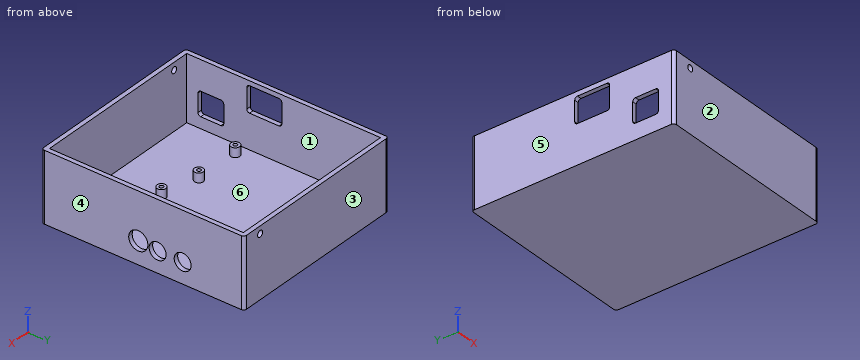
```python
from build123d import *

# Parameters (mm, degrees)
FLOOR_2P4MM_DEPTH                         = 2.4
SIX_PCB_SUPPORTS_5MM_START                = 2.4
SKETCH_2_R                                = 2.4
SIX_PCB_SUPPORTS_5MM_DEPTH                = 5
INTEGRAL_FRONT_REAR_AND_SIDE_WALLS_START  = 2.4
SKETCH_3_W                                = 94.1
SKETCH_3_H                                = 105.2
INTEGRAL_FRONT_REAR_AND_SIDE_WALLS_DEPTH  = 35.2
SIX_BLIND_M2P5_STANDOFF_PILOTS_DEPTH      = 2.05
SIX_BLIND_M2P5_STANDOFF_PILOTS_DEPTH_BACK = 2.05
SIX_BLIND_M2P5_STANDOFF_PILOTS_START      = 5.35
SKETCH_4_R                                = 1.05
SIDE_LID_SCREW_1_DEPTH                    = 1.25
SIDE_LID_SCREW_1_DEPTH_BACK               = 1.25
SIDE_LID_SCREW_1_START                    = -8.3
SKETCH_5_R                                = 1.7
SIDE_LID_SCREW_2_DEPTH                    = 1.25
SIDE_LID_SCREW_2_DEPTH_BACK               = 1.25
SIDE_LID_SCREW_2_START                    = 99.3
SKETCH_6_R                                = 1.7
FRONT_AUDIO_ACCESS_DEPTH                  = 1.25
FRONT_AUDIO_ACCESS_DEPTH_BACK             = 1.25
FRONT_AUDIO_ACCESS_START                  = 93.7
SKETCH_7_R                                = 5.2
SKETCH_7_R_2                              = 4.6
REAR_DC_AND_USB_ACCESS_DEPTH              = 1.25
REAR_DC_AND_USB_ACCESS_DEPTH_BACK         = 1.25
REAR_DC_AND_USB_ACCESS_START              = -2.8


with BuildPart() as part:
    # 草图1 → Floor_2p4mm (new body)
    with BuildSketch(Plane.XY):
        with BuildLine():
            Line((-2.5, -9.5), (93.4, -9.5))
            ThreePointArc((93.4, -9.5), (94.460660172, -9.060660172), (94.9, -8))
            Line((94.9, -8), (94.9, 99))
            ThreePointArc((94.9, 99), (94.460660172, 100.060660172), (93.4, 100.5))
            Line((93.4, 100.5), (-2.5, 100.5))
            ThreePointArc((-2.5, 100.5), (-3.560660172, 100.060660172), (-4, 99))
            Line((-4, 99), (-4, -8))
            ThreePointArc((-4, -8), (-3.560660172, -9.060660172), (-2.5, -9.5))
        make_face()
    extrude(amount=FLOOR_2P4MM_DEPTH)

    # 草图2 → Six_PCB_supports_5mm (add)
    with BuildSketch(Plane.XY.offset(SIX_PCB_SUPPORTS_5MM_START)):
        with Locations((5, 24.5)):
            Circle(SKETCH_2_R)
        with Locations((5, 88)):
            Circle(SKETCH_2_R)
        with Locations((30, 24.5)):
            Circle(SKETCH_2_R)
        with Locations((30, 88)):
            Circle(SKETCH_2_R)
        with Locations((78, 12)):
            Circle(SKETCH_2_R)
        with Locations((50, 20)):
            Circle(SKETCH_2_R)
    extrude(amount=SIX_PCB_SUPPORTS_5MM_DEPTH)

    # 草图3 → Integral_front_rear_and_side_walls (add)
    with BuildSketch(Plane.XY.offset(INTEGRAL_FRONT_REAR_AND_SIDE_WALLS_START)):
        with BuildLine():
            Line((-2.5, -9.5), (93.4, -9.5))
            ThreePointArc((93.4, -9.5), (94.460660172, -9.060660172), (94.9, -8))
            Line((94.9, -8), (94.9, 99))
            ThreePointArc((94.9, 99), (94.460660172, 100.060660172), (93.4, 100.5))
            Line((93.4, 100.5), (-2.5, 100.5))
            ThreePointArc((-2.5, 100.5), (-3.560660172, 100.060660172), (-4, 99))
            Line((-4, 99), (-4, -8))
            ThreePointArc((-4, -8), (-3.560660172, -9.060660172), (-2.5, -9.5))
        make_face()
        with Locations((45.45, 45.5)):
            Rectangle(SKETCH_3_W, SKETCH_3_H, mode=Mode.SUBTRACT)
    extrude(amount=INTEGRAL_FRONT_REAR_AND_SIDE_WALLS_DEPTH)

    # 草图4 → Six_blind_M2p5_standoff_pilots (cut, two sides: drawn at the far end of the back side and taken through both)
    with BuildSketch(Plane.XY.offset(SIX_BLIND_M2P5_STANDOFF_PILOTS_START - SIX_BLIND_M2P5_STANDOFF_PILOTS_DEPTH_BACK)):
        with Locations((5, 24.5)):
            Circle(SKETCH_4_R)
        with Locations((5, 88)):
            Circle(SKETCH_4_R)
        with Locations((30, 24.5)):
            Circle(SKETCH_4_R)
        with Locations((30, 88)):
            Circle(SKETCH_4_R)
        with Locations((78, 12)):
            Circle(SKETCH_4_R)
        with Locations((50, 20)):
            Circle(SKETCH_4_R)
    extrude(amount=SIX_BLIND_M2P5_STANDOFF_PILOTS_DEPTH + SIX_BLIND_M2P5_STANDOFF_PILOTS_DEPTH_BACK, mode=Mode.SUBTRACT)

    # 草图5 → Side_lid_screw_1 (cut, two sides: drawn at the far end of the back side and taken through both)
    with BuildSketch(Plane(origin=(0, 0, 0), x_dir=(1, 0, 0), z_dir=(0, 1, 0)).offset(SIDE_LID_SCREW_1_START - SIDE_LID_SCREW_1_DEPTH_BACK)):
        with Locations(Location((7, -33.6, 0), (0, 0, 270))):
            Circle(SKETCH_5_R)
    extrude(amount=SIDE_LID_SCREW_1_DEPTH + SIDE_LID_SCREW_1_DEPTH_BACK, mode=Mode.SUBTRACT)

    # 草图6 → Side_lid_screw_2 (cut, two sides: drawn at the far end of the back side and taken through both)
    with BuildSketch(Plane(origin=(0, 0, 0), x_dir=(1, 0, 0), z_dir=(0, 1, 0)).offset(SIDE_LID_SCREW_2_START - SIDE_LID_SCREW_2_DEPTH_BACK)):
        with Locations(Location((84, -33.6, 0), (0, 0, 90))):
            Circle(SKETCH_6_R)
    extrude(amount=SIDE_LID_SCREW_2_DEPTH + SIDE_LID_SCREW_2_DEPTH_BACK, mode=Mode.SUBTRACT)

    # 草图7 → Front_audio_access (cut, two sides: drawn at the far end of the back side and taken through both)
    with BuildSketch(Plane(origin=(0, 0, 0), x_dir=(0, 0, -1), z_dir=(1, 0, 0)).offset(FRONT_AUDIO_ACCESS_START - FRONT_AUDIO_ACCESS_DEPTH_BACK)):
        with Locations(Location((-12.25, 43.0009, 0), (0, 0, 180))):
            Circle(SKETCH_7_R)
        with Locations(Location((-11.25, 53.5, 0), (0, 0, 180))):
            Circle(SKETCH_7_R_2)
        with Locations(Location((-11.25, 67.1, 0), (0, 0, 180))):
            Circle(SKETCH_7_R_2)
    extrude(amount=FRONT_AUDIO_ACCESS_DEPTH + FRONT_AUDIO_ACCESS_DEPTH_BACK, mode=Mode.SUBTRACT)

    # 草图8 → Rear_DC_and_USB_access (cut, two sides: drawn at the far end of the back side and taken through both)
    with BuildSketch(Plane(origin=(0, 0, 0), x_dir=(0, 0, -1), z_dir=(1, 0, 0)).offset(REAR_DC_AND_USB_ACCESS_START - REAR_DC_AND_USB_ACCESS_DEPTH_BACK)):
        with BuildLine():
            Line((-8.5, 0.5), (-8.5, 11.5))
            ThreePointArc((-8.5, 11.5), (-8.939339828, 12.560660172), (-10, 13))
            Line((-10, 13), (-20, 13))
            ThreePointArc((-20, 13), (-21.060660172, 12.560660172), (-21.5, 11.5))
            Line((-21.5, 11.5), (-21.5, 0.5))
            ThreePointArc((-21.5, 0.5), (-21.060660172, -0.560660172), (-20, -1))
            Line((-20, -1), (-10, -1))
            ThreePointArc((-10, -1), (-8.939339828, -0.560660172), (-8.5, 0.5))
        make_face()
        with BuildLine():
            Line((-21.1, 27), (-21.1, 43))
            ThreePointArc((-21.1, 43), (-21.539339828, 44.060660172), (-22.6, 44.5))
            Line((-22.6, 44.5), (-33.6, 44.5))
            ThreePointArc((-33.6, 44.5), (-34.660660172, 44.060660172), (-35.1, 43))
            Line((-35.1, 43), (-35.1, 27))
            ThreePointArc((-35.1, 27), (-34.660660172, 25.939339828), (-33.6, 25.5))
            Line((-33.6, 25.5), (-22.6, 25.5))
            ThreePointArc((-22.6, 25.5), (-21.539339828, 25.939339828), (-21.1, 27))
        make_face()
    extrude(amount=REAR_DC_AND_USB_ACCESS_DEPTH + REAR_DC_AND_USB_ACCESS_DEPTH_BACK, mode=Mode.SUBTRACT)


solid = part.part
```
Here's how the part is built. I have some questions about the finished solid (model axes, mm). Face numbers are marked on the shaded views. A direction names the side the tool comes from. Round coordinates to 2 decimals unless told otherwise and drop trailing zeros. Loops run counter-clockwise (first coordinate to the right, second up) from the corner with the lowest first, then second, coordinate; pieces in that order, holes last.
1. Suppose I cut it at C-C, the plane x = 71.5. Please give me the cut outline in (y, z), and give its area (3 significant figures).
Answers:
outline: (-9.5, 0) - (100.5, 0) - (100.5, 37.6) - (98.1, 37.6) - (98.1, 2.4) - (-7.1, 2.4) - (-7.1, 37.6) - (-9.5, 37.6) - close
area: 433 mm2
2. If I drill on probe 1 along Z at (x, y) = (94, 67); probe 2 along X at (y, z) = (92.5, 29); probe 3 along Y at (x, z) = (89.5, 24), over which ranges is the centre line in solid material (lowest first)?
Answers:
probe 1: z = 0 to 6.65, 15.85 to 37.6
probe 2: x = -4 to -1.6, 92.5 to 94.9
probe 3: y = -9.5 to -7.1, 98.1 to 100.5
3. Suppose I cut it at A-A, the plane x = 84. Please give me the cut outline in (y, z), and give its area (3 significant figures).
Answers:
outline: (-9.5, 0) - (100.5, 0) - (100.5, 31.9) - (98.1, 31.9) - (98.1, 2.4) - (-7.1, 2.4) - (-7.1, 37.6) - (-9.5, 37.6) - close; (98.1, 35.3) - (100.5, 35.3) - (100.5, 37.6) - (98.1, 37.6) - close
area: 425 mm2
4. Suppose I cut it at B-B, the plane z = 13. Please give me the cut outline in (x, y), and give its area (3 significant figures).
Answers:
outline: (-4, -8) arc R1.5 ccw to (-2.5, -9.5) - (93.4, -9.5) arc R1.5 ccw to (94.9, -8) - (94.9, 37.86) - (92.5, 37.86) - (92.5, -7.1) - (-1.6, -7.1) - (-1.6, -1) - (-4, -1) - close; (-4, 13) - (-1.6, 13) - (-1.6, 98.1) - (92.5, 98.1) - (92.5, 71.35) - (94.9, 71.35) - (94.9, 99) arc R1.5 ccw to (93.4, 100.5) - (-2.5, 100.5) arc R1.5 ccw to (-4, 99) - close; (92.5, 48.15) - (94.9, 48.15) - (94.9, 49.25) - (92.5, 49.25) - close; (92.5, 57.75) - (94.9, 57.75) - (94.9, 62.85) - (92.5, 62.85) - close
area: 879 mm2
5. For the marked faces 5 and 6, which set-ups out of +Z, -Z, +X, -X, +Y, -Y let a thin tool reach every point of the face, with its end or its side?
Answers:
face 5: +Z, -Z, -X, +Y, -Y
face 6: +Z
6. Will these pins go through, and if not, where does the flat tip stop? pin 1 (10 mm diameter, centred on x = 34, y = 41, fed in from +Z); pin 2 (1.7 mm diameter, centred on x = 4.5, y = 88, fed in from +Z); pin 3 (0.6 mm diameter, centred on x = 30, y = 24.5, fed in from +Z).
Answers:
pin 1: stops at z = 2.4
pin 2: stops at z = 7.4
pin 3: stops at z = 3.3
7. Thinking about a two-plate mould opening in Y: for the marked faces 1, 2, 3 and 4, which applies, released by +Y, released by -Y, zero draft, split by the parting line, or undercut?
Answers:
face 1: undercut
face 2: released by -Y
face 3: released by +Y
face 4: zero draft
